Here's the drawing with two shaded views (mm, measured from the low corner). I have some questions. A direction names the side the tool comes from. Give positions to 0.01 mm unless a question says otherwise; leave off trailing zeros. Write each loop counter-clockwise with the first axis right and the second up, starting at its lowest first coordinate (ties: lowest second). Pieces come first, ordered by that corner, then holes.
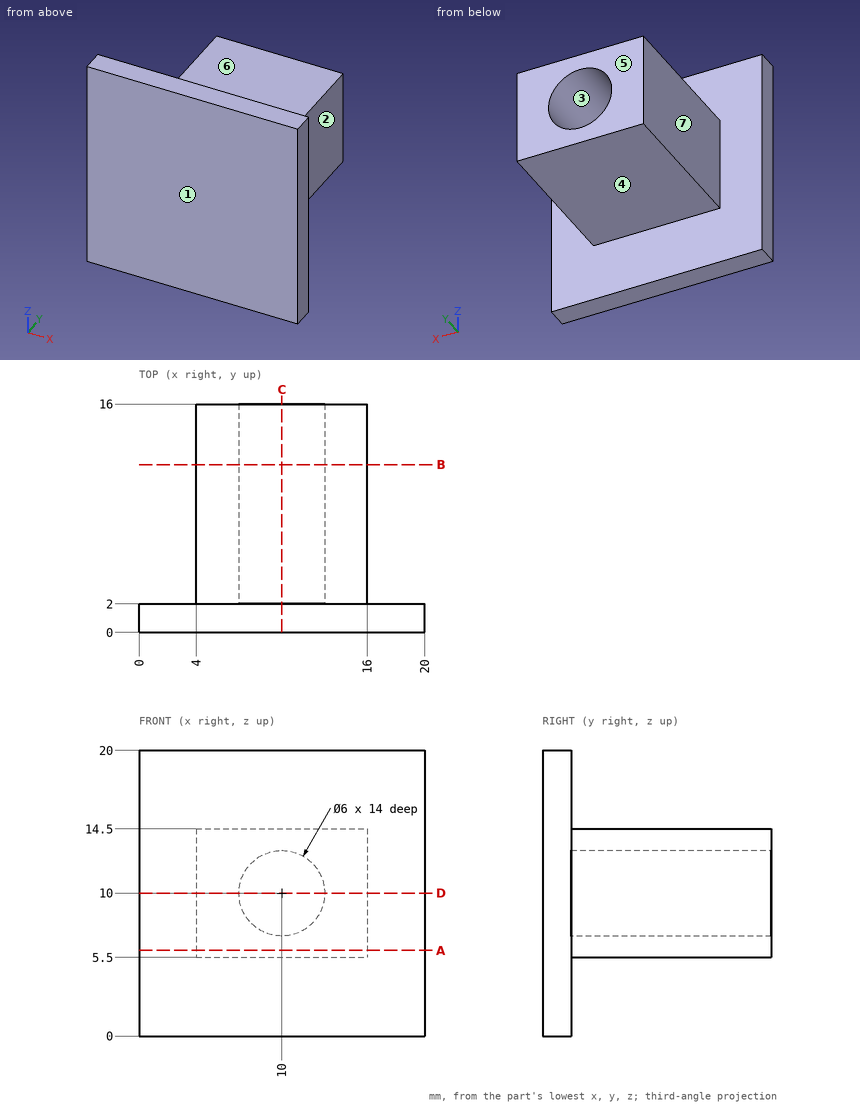
(1) For the marked faces 4, 5, 6 and 7, which set-ups out of +Z, -Z, +X, -X, +Y, -Y let a thin tool reach every point of the face, with its end or its side?
Returned:
face 4: -Z, +X, -X, +Y
face 5: +Z, -Z, +X, -X, +Y
face 6: +Z, +X, -X, +Y
face 7: +Z, -Z, -X, +Y
(2) Imagine slicing it at A-A, the plane z = 6. Write out the boundary of the cut face in (x, y), plus the area to 3 significant figures.
Returned:
outline: (0, 0) - (20, 0) - (20, 2) - (16, 2) - (16, 16) - (4, 16) - (4, 2) - (0, 2) - close
area: 208 mm2
(3) Imagine slicing it at B-B, the plane y = 11.75. Write out the boundary of the cut face in (x, z).
Returned:
outline: (4, 5.5) - (16, 5.5) - (16, 14.5) - (4, 14.5) - close; hole circle Ø6 at (10, 10)
(4) Will these pins go through, and if not, where does the flat tip stop? P1, Ø9.5, axis at x = 7, y = 6.5, coming from the +Z side; P2, Ø7, axis at y = 7, z = 12, coming from the +X side; P3, Ø2.5, axis at y = 12, z = 8.5, coming from the -X side; P4, Ø9.5, axis at x = 7, y = 9, coming from the -Z side.
Returned:
P1: stops at z = 20
P2: stops at x = 16
P3: stops at x = 4
P4: stops at z = 5.5
(5) Imagine slicing it at C-C, the plane x = 10. Write out the boundary of the cut face in (y, z).
Returned:
outline: (0, 0) - (2, 0) - (2, 5.5) - (16, 5.5) - (16, 7) - (2, 7) - (2, 13) - (16, 13) - (16, 14.5) - (2, 14.5) - (2, 20) - (0, 20) - close
(6) Imagine slicing it at D-D, the plane z = 10. Write out the boundary of the cut face in (x, y), plus the area to 3 significant figures.
Returned:
outline: (0, 0) - (20, 0) - (20, 2) - (16, 2) - (16, 16) - (13, 16) - (13, 2) - (7, 2) - (7, 16) - (4, 16) - (4, 2) - (0, 2) - close
area: 124 mm2
(7) If I drill on L1, parallel to X at y = 9.75, z = 10; L2, parallel to Y at x = 17.25, z = 4.5; L3, parallel to Z at x = 6.75, y = 8, over which ranges is the centre line in solid material (lowest first)?
Returned:
L1: x = 4 to 7, 13 to 16
L2: y = 0 to 2
L3: z = 5.5 to 14.5
(8) If we mould it in two halves opening along X, with no side actions, what happens to the marked faces 1, 2 and 3? For each: +X half, -X half, draft (parallel to the pull), parting line (faces both ways), or undercut.
Returned:
face 1: draft
face 2: +X half
face 3: undercut
